Build history of the part. All positions in model axes, mm. A direction names the side the tool comes from. Round coordinates to 2 decimals unless told otherwise and drop trailing zeros. Order: outer loops, then holes, each group sorted by start corner. A loop starts at its lowest first (then second) coordinate and runs counter-clockwise, first axis right, second up. Notation, with made-up numbers: M 83,7 L 106,7 A9 cw 106,20 Z; hole C 43,49.25 d11. An arc over 180 degrees is marked long. One line per item, written item: value. Start each with the question number.
Item 1: Band-saw the part on C-C, the plane x = -33. Write the cut outline in (y, z) (3 decimals), then the cut area to 3 significant figures.
Item 2: Two-plate mould, pull along X, no slides. Class faces 1 (the flat face through (-37.793, 0.889, 14.488)), 2 (the flat face through (6.35, -1, 2)), 3 (the flat face through (-6.35, -1, 2)), 4 (the flat face through (8, 1, 0)): +X half, -X half, draft (parallel to the pull), parting line (faces both ways), or undercut.
Item 3: Pin check, flat tips, straight feed: pin 1 (12 mm diameter, centred on y = -8, z = 11, fed in from +X); pin 2 (3.5 mm diameter, centred on y = 14, z = 1, fed in from +X); pin 3 (3 mm diameter, centred on x = -32.5, y = 0.5, fed in from +Z). Stop position of each tip, or through.
Item 4: Band-saw the part on D-D, the plane z = 17.5. Write the cut outline in (x, y) (3 decimals), then the cut area to 3 significant figures.
Item 5: Band-saw the part on A-A, the plane y = 50. Write the cut outline in (x, z) (3 decimals).
Item 6: Probe L1, parallel to Y at x = -50, z = 22.25 (3 decimals); L2, parallel to Y at x = -15, z = 21 (3 decimals); L3, parallel to X at y = 38, z = 26.25. List the from-to ranges inside material, lowest first.
Item 7: Tool access for faces 5 (the flat face through (-34.39, 0.84, 15.7)), 6 (the flat face through (0, 57.15, 2)), 7 (the flat face through (60, 0, 28.575)): list every direction of +Z, -Z, +X, -X, +Y, -Y with a clear straight run to the whole face (end or side of a thin tool).
Item 8: Band-saw the part on B-B, the plane y = -11. Write the cut outline in (x, z) (3 decimals), then the cut area to 3 significant figures.
```python
from build123d import *

# Parameters (mm, degrees)
F0_W          = 25.4
F0_H          = 127
F0_W_2        = 12.7
F0_H_2        = 114.3
F1_DEPTH      = 3.175
F3_DEPTH      = 63.5
F3_DEPTH_BACK = 63.5
F7_DEPTH      = 3.175
F9_DEPTH      = 3.175
F10_W         = 31.6360226281
F10_H         = 28.575
F11_DEPTH     = 62.1943518263


with BuildPart() as f1:
    # F0 (on Top) → F1 (new body)
    with BuildSketch(Plane.XY):
        Rectangle(F0_W, F0_H)
        Rectangle(F0_W_2, F0_H_2, mode=Mode.SUBTRACT)
    extrude(amount=F1_DEPTH)

    # F2 (on Front) → F3 (join, two sides)
    with BuildSketch(Plane.XZ) as f3_sk:
        Polygon((56.6940905122, 28.575), (12.7, 3.175), (18.199261314, 3.175), (62.1933518263, 28.575), align=None)
        Polygon((18.199261314, 3.175), (12.7, 3.175), (12.7, 0), align=None)
        Polygon((-12.7, 3.175), (-56.6940905122, 28.575), (-62.1933518263, 28.575), (-12.7, 0), align=None)
    extrude(amount=F3_DEPTH)
    extrude(f3_sk.sketch, amount=-F3_DEPTH_BACK)

    # F6 (on offset) → F7 (join)
    with BuildSketch(Plane.XZ.offset(63.5)):
        Polygon((62.1933518263, 28.575), (-62.1933518263, 28.575), (-12.7, 0), (12.7, 0), align=None)
    extrude(amount=-F7_DEPTH)

    # F8 (on offset) → F9 (join)
    with BuildSketch(Plane.XZ.offset(-63.5)):
        Polygon((62.1933518263, 28.575), (-62.1933518263, 28.575), (-12.7, 0), (12.7, 0), align=None)
    extrude(amount=F9_DEPTH)

    # F10 (on face) → F11 (cut, through all)
    with BuildSketch(Plane(origin=(-3.175, 0, -5.499261314), x_dir=(0.8660254038, 0, -0.5), z_dir=(-0.5, 0, -0.8660254038))):
        with Locations((-41.218011314, 39.6875)):
            Rectangle(F10_W, F10_H)
        with Locations((-41.218011314, -39.6875)):
            Rectangle(F10_W, F10_H)
    extrude(amount=-F11_DEPTH, mode=Mode.SUBTRACT)


solid = f1.part
```
Output:
1. outline: M -63.5,11.72 L -53.975,11.72 L -53.975,14.895 L -60.325,14.895 L -60.325,28.575 L -63.5,28.575 Z; M -25.4,11.72 L 25.4,11.72 L 25.4,14.895 L -25.4,14.895 Z; M 53.975,11.72 L 63.5,11.72 L 63.5,28.575 L 60.325,28.575 L 60.325,14.895 L 53.975,14.895 Z
1. area: 309 mm²
2. face 1: -X half
2. face 2: undercut
2. face 3: undercut
2. face 4: draft
3. pin 1: stops at x = 42.14
3. pin 2: stops at x = 17.46
3. pin 3: stops at z = 15.47
4. outline: M -43.011,-63.5 L 43.011,-63.5 L 43.011,63.5 L -43.011,63.5 L -43.011,53.975 L -37.512,53.975 L -37.512,60.325 L 37.512,60.325 L 37.512,-60.325 L -37.512,-60.325 L -37.512,-53.975 L -43.011,-53.975 Z; M -43.011,-25.4 L -37.512,-25.4 L -37.512,25.4 L -43.011,25.4 Z
4. area: 1,560 mm²
5. outline: M -62.193,28.575 L -52.57,23.019 L -51.195,25.4 L -56.694,28.575 Z; M -25.172,7.201 L -12.7,0 L -6.35,0 L -6.35,3.175 L -12.7,3.175 L -23.797,9.582 Z; M 6.35,0 L 12.7,0 L 62.193,28.575 L 56.694,28.575 L 12.7,3.175 L 6.35,3.175 Z
6. L1: y = -63.5 to -53.975, -25.4 to 25.4, 53.975 to 63.5
6. L2: y = -63.5 to -60.325, 60.325 to 63.5
6. L3: x = -58.17 to -52.67, 52.67 to 58.17
7. face 5: +Z
7. face 6: +Z, -Z
7. face 7: +Z, +X, -X, +Y, -Y
8. outline: M -62.193,28.575 L -12.7,0 L -6.35,0 L -6.35,3.175 L -12.7,3.175 L -56.694,28.575 Z; M 6.35,0 L 12.7,0 L 62.193,28.575 L 56.694,28.575 L 12.7,3.175 L 6.35,3.175 Z
8. area: 337 mm²
